Can you work these out from the model? Positions are in its coordinate system, mm. Face numbers are marked on the shaded views. Coordinates: 2 decimals unless noted, no trailing zeros. Order: outer loops, then holes, each group sorted by start corner. A loop starts at its lowest first (then second) coordinate and runs counter-clockwise, first axis right, second up. Notation, with made-up numbers: (-16.75, 31.5) - (22.25, 31.5) arc R26 ccw to (22.25, 52.5) - close; hole circle Ø2 at (67, 44.5). An arc over 180 degrees is marked (long way). Return JSON: item names as keys, results as strings. Group by question number.
1) For pin 1 Ø7 at (x, y) = (14.5, 5.5) entering from +Z, with a flat end and sliding along its axis, tell me the tip position at first contact or that it passes through.
2) Imagine slicing it at A-A (z = 8.5). Write out the boundary of the cut face in (x, y).
3) If I drill on line 1 along Y through (x, z) = (21.5, 7.5); line 2 along X through (y, z) = (65, 12); line 3 along Y through (x, z) = (18, 2.5), over which ranges is the centre line in solid material (lowest first)?
4) If we mould it in two halves opening along X, with no side actions, what happens to the marked faces 1, 2 and 3? For each: pulls with the +X half, pulls with the -X half, needs draft (parallel to the pull), parting line crosses it, or undercut.
5) Imagine slicing it at B-B (x = 17.5). Give the number of separate pieces and of enclosed holes in the cut face, and give its area (3 significant figures).
6) Imagine slicing it at C-C (z = 3.5). Write out the boundary of the cut face in (x, y).
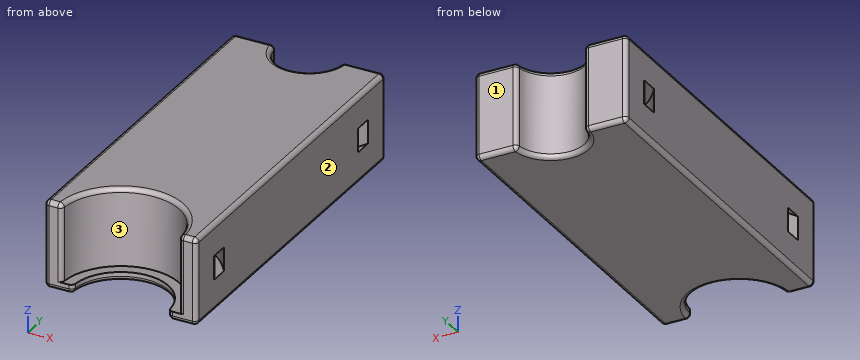
```python
from build123d import *

# Parameters (mm, degrees)
PAD_DEPTH    = 20
SKETCH002_W  = 2
SKETCH002_H  = 5.5
SKETCH004_W  = 2
SKETCH004_H  = 5.5
PAD001_DEPTH = 2
FILLET_R     = 1


with BuildPart() as part:
    # Sketch → Pad (new body)
    with BuildSketch(Plane.XY):
        with BuildLine():
            Line((0, 0), (4, 0))
            ThreePointArc((31, 0), (17.5, 13.5), (4, 0))
            Line((31, 0), (35, 0))
            Line((35, 0), (35, 80))
            Line((35, 80), (25.25, 80))
            ThreePointArc((9.75, 80), (17.5, 72.25), (25.25, 80))
            Line((9.75, 80), (0, 80))
            Line((0, 80), (0, 0))
        make_face()
    extrude(amount=PAD_DEPTH)

    # SubtractivePipe: sweep along a path in Sketch001
    with BuildLine(Plane.XY.offset(10)) as subtractivepipe_path:
        CenterArc((17.5, 0), 20, 0, 360)
    # Sketch002 → SubtractivePipe (sweep, cut)
    with BuildSketch(Plane.XZ):
        with Locations((37.5, 10)):
            Rectangle(SKETCH002_W, SKETCH002_H)
    sweep(path=subtractivepipe_path.line, mode=Mode.SUBTRACT)

    # SubtractivePipe001: sweep along a path in Sketch003
    with BuildLine(Plane.XY.offset(10)) as subtractivepipe001_path:
        CenterArc((17.5, 80), 20, 0, 360)
    # Sketch004 → SubtractivePipe001 (sweep, cut)
    with BuildSketch(Plane.XZ.offset(-80)):
        with Locations((37.5, 10)):
            Rectangle(SKETCH004_W, SKETCH004_H)
    sweep(path=subtractivepipe001_path.line, mode=Mode.SUBTRACT)

    # Sketch005 → Pad001 (join)
    with BuildSketch(Plane.XY):
        with BuildLine():
            ThreePointArc((28.5, 0), (17.5, 11), (6.5, 0))
            Line((6.5, 0), (4, 0))
            ThreePointArc((31, 0), (17.5, 13.5), (4, 0))
            Line((31, 0), (28.5, 0))
        make_face()
    extrude(amount=PAD001_DEPTH)

    # Fillet
    fillet_edges = [part.edges().sort_by_distance(p)[0] for p in [
        (0, 40, 20),
        (35, 40, 20),
        (2, 0, 20),
        (17.5, 13.5, 20),
        (33, 0, 20),
        (4, 0, 11),
        (0, 0, 10),
        (31, 0, 11),
        (35, 0, 10),
        (3.25, 0, 0),
        (31.75, 0, 0),
        (35, 40, 0),
        (17.5, 11, 0),
        (0, 40, 0),
        (4.875, 80, 0),
        (17.5, 72.25, 0),
        (30.125, 80, 0),
        (35, 80, 10),
        (25.25, 80, 10),
        (9.75, 80, 10),
        (30.125, 80, 20),
        (4.875, 80, 20),
        (17.5, 72.25, 20),
        (0, 80, 10),
        (28.5, 0, 1),
        (6.5, 0, 1),
    ]]
    fillet(fillet_edges, radius=FILLET_R)


solid = part.part
```
Calculated:
{
 "1": {"pin 1": "through"},
 "2": {"outline": "(0, 1) arc R1 ccw to (1, 0) - (3.03, 0) arc R1 ccw to (4.03, 0.93) arc R13.5 cw to (30.97, 0.93) arc R1 ccw to (31.97, 0) - (34, 0) arc R1 ccw to (35, 1) - (35, 7.4) arc R19 ccw to (0, 7.4) - close; (0, 11.61) arc R21 cw to (35, 11.61) - (35, 68.39) arc R21 cw to (0, 68.39) - close; (0, 72.6) arc R19 ccw to (35, 72.6) - (35, 79) arc R1 ccw to (34, 80) - (26.19, 80) arc R1 ccw to (25.2, 79.11) arc R7.75 cw to (9.8, 79.11) arc R1 ccw to (8.81, 80) - (1, 80) arc R1 ccw to (0, 79) - close"},
 "3": {"line 1": "12.89 to 18.57, 20.62 to 59.38, 61.43 to 73.36", "line 2": "0 to 2.8, 5.84 to 29.16, 32.2 to 35", "line 3": "13.49 to 72.27"},
 "4": {"face 1": "needs draft", "face 2": "pulls with the +X half", "face 3": "undercut"},
 "5": {"separate pieces": "1", "enclosed holes": "2", "area": "1,160 mm2"},
 "6": {"outline": "(0, 1) arc R1 ccw to (1, 0) - (3.03, 0) arc R1 ccw to (4.03, 0.93) arc R13.5 cw to (30.97, 0.93) arc R1 ccw to (31.97, 0) - (34, 0) arc R1 ccw to (35, 1) - (35, 79) arc R1 ccw to (34, 80) - (26.19, 80) arc R1 ccw to (25.2, 79.11) arc R7.75 cw to (9.8, 79.11) arc R1 ccw to (8.81, 80) - (1, 80) arc R1 ccw to (0, 79) - close"}
}
